Geometry: final body of the model. Coordinates: model frame, mm. A direction names the side the tool comes from. Give positions to 0.01 mm unless a question says otherwise; leave off trailing zeros. Order: outer loops, then holes, each group sorted by start corner. A loop starts at its lowest first (then second) coordinate and runs counter-clockwise, first axis right, second up. Notation, with made-up numbers: (44, 27) - (97, 27) arc R13 ccw to (97, 42) - close; hole circle Ø1 at (3, -10.75). An arc over 180 degrees is marked (long way). Use one line per item in the form item = value.
from build123d import *

# Parameters (mm, degrees)
BOSS_EXTRUDE1_DEPTH = 5.08
SKETCH2_R           = 1.778
CUT_EXTRUDE1_DEPTH  = 55.120480412
SKETCH3_W           = 43.18
SKETCH3_H           = 20.32
CUT_EXTRUDE2_DEPTH  = 55.120480412
SKETCH10_R          = 1.524
CUT_EXTRUDE3_DEPTH  = 55.120480412
SKETCH11_W          = 7.62
SKETCH11_H          = 2.54
CUT_EXTRUDE4_DEPTH  = 55.120480412
CUT_EXTRUDE5_DEPTH  = 55.120480412
SKETCH14_R          = 1.905
CUT_EXTRUDE6_DEPTH  = 55.120480412
CHAMFER1_SIZE       = 16.51
CHAMFER3_SIZE       = 16.51
FILLET1_R           = 12.7
FILLET2_R           = 12.7
SKETCH15_W          = 6.35
SKETCH15_H          = 25.4
CUT_EXTRUDE7_DEPTH  = 55.120480412
SKETCH18_W          = 25.4
SKETCH18_H          = 12.7
BOSS_EXTRUDE3_DEPTH = 5.08
SKETCH19_R          = 0.889
CUT_EXTRUDE9_DEPTH  = 69.814783295
FILLET4_R           = 6.35
SKETCH20_W          = 25.4
SKETCH20_H          = 2.54
CUT_EXTRUDE10_DEPTH = 69.814783351
CHAMFER4_SIZE       = 7.62
CHAMFER4_SIZE2      = 4.399409051
FILLET5_R           = 6.35
FILLET6_R           = 6.35


with BuildPart() as part:
    # Sketch1 → Boss-Extrude1 (new body)
    with BuildSketch(Plane(origin=(0, 0, 0), x_dir=(1, 0, 0), z_dir=(0, 1, 0))):
        Polygon((-38.1, -12.7), (-38.1, 38.1), (38.1, 38.1), (38.1, -12.7), (19.05, -12.7), (19.05, -38.1), (-19.05, -38.1), (-19.05, -12.7), align=None)
    extrude(amount=BOSS_EXTRUDE1_DEPTH)

    # Sketch2 → Cut-Extrude1 (cut, through all)
    with BuildSketch(Plane(origin=(0, 5.08, 0), x_dir=(1, 0, 0), z_dir=(0, 1, 0))):
        with Locations(Location((-22.225, 29.972, 0), (0, 0, 270))):
            Circle(SKETCH2_R)
        with Locations(Location((22.225, 29.972, 0), (0, 0, 90))):
            Circle(SKETCH2_R)
    extrude(amount=-CUT_EXTRUDE1_DEPTH, mode=Mode.SUBTRACT)

    # Sketch3 → Cut-Extrude2 (cut, through all)
    with BuildSketch(Plane(origin=(0, 5.08, 0), x_dir=(1, 0, 0), z_dir=(0, 1, 0))):
        with Locations((0, 9.652)):
            Rectangle(SKETCH3_W, SKETCH3_H)
    extrude(amount=-CUT_EXTRUDE2_DEPTH, mode=Mode.SUBTRACT)

    # Sketch10 → Cut-Extrude3 (cut, through all)
    with BuildSketch(Plane.XZ):
        with Locations(Location((25.4, -14.859, 0), (0, 0, 270))):
            Circle(SKETCH10_R)
        with Locations(Location((25.4, -4.445, 0), (0, 0, 90))):
            Circle(SKETCH10_R)
        with Locations(Location((-25.4, -14.859, 0), (0, 0, 90))):
            Circle(SKETCH10_R)
        with Locations(Location((-25.4, -4.445, 0), (0, 0, 270))):
            Circle(SKETCH10_R)
    extrude(amount=-CUT_EXTRUDE3_DEPTH, mode=Mode.SUBTRACT)

    # Sketch11 → Cut-Extrude4 (cut, through all)
    with BuildSketch(Plane.XZ):
        with Locations((25.4, -9.652)):
            Rectangle(SKETCH11_W, SKETCH11_H)
        with Locations((-25.4, -9.652)):
            Rectangle(SKETCH11_W, SKETCH11_H)
    extrude(amount=-CUT_EXTRUDE4_DEPTH, mode=Mode.SUBTRACT)

    # Sketch12 → Cut-Extrude5 (cut, through all)
    with BuildSketch(Plane.XZ):
        Polygon((22.225, -38.1), (0, -30.48), (-22.225, -38.1), align=None)
    extrude(amount=-CUT_EXTRUDE5_DEPTH, mode=Mode.SUBTRACT)

    # Sketch14 → Cut-Extrude6 (cut, through all)
    with BuildSketch(Plane.XZ):
        with Locations(Location((31.75, 3.048, 0), (0, 0, 270))):
            Circle(SKETCH14_R)
        with Locations(Location((31.75, -22.352, 0), (0, 0, 90))):
            Circle(SKETCH14_R)
        with Locations(Location((-31.75, 3.048, 0), (0, 0, 90))):
            Circle(SKETCH14_R)
        with Locations(Location((-31.75, -22.352, 0), (0, 0, 270))):
            Circle(SKETCH14_R)
    extrude(amount=-CUT_EXTRUDE6_DEPTH, mode=Mode.SUBTRACT)

    # Chamfer1
    # the kernel refuses this chamfer: 16.51 mm, written as the material it takes off along each edge
    with BuildSketch(Plane(origin=(38.1, -42.458486131, -38.1), x_dir=(0.027495876610586233, 0, 0.9996219169112966), z_dir=(0, 1, 0))) as chamfer1_piece_1:
        Polygon((CHAMFER1_SIZE * 0.999621916911, -CHAMFER1_SIZE * 0.0274958766106), (-CHAMFER1_SIZE * 0.0274958766106, -CHAMFER1_SIZE * 0.999621916911), (0, 0), align=None)
    extrude(amount=89.996972263, mode=Mode.SUBTRACT)

    # Chamfer3
    # the kernel refuses this chamfer: 16.51 mm, written as the material it takes off along each edge
    with BuildSketch(Plane(origin=(-38.1, -42.458486131, -38.1), x_dir=(-0.02749587661058624, 0, 0.9996219169112966), z_dir=(0, 1, 0))) as chamfer3_piece_1:
        Polygon((CHAMFER3_SIZE * 0.999621916911, CHAMFER3_SIZE * 0.0274958766106), (-CHAMFER3_SIZE * 0.0274958766106, CHAMFER3_SIZE * 0.999621916911), (0, 0), align=None)
    extrude(amount=89.996972263, mode=Mode.SUBTRACT)

    # Fillet1
    fillet1_edges = [part.edges().sort_by_distance(p)[0] for p in [
        (21.75212766, 2.54, -37.93787234),
        (-21.75212766, 2.54, -37.93787234),
    ]]
    fillet(fillet1_edges, radius=FILLET1_R)

    # Fillet2
    fillet2_edges = [part.edges().sort_by_distance(p)[0] for p in [
        (38.1, 2.54, 12.7),
        (-38.1, 2.54, 12.7),
    ]]
    fillet(fillet2_edges, radius=FILLET2_R)

    # Sketch15 → Cut-Extrude7 (cut, through all)
    with BuildSketch(Plane.XZ):
        with Locations((15.875, 25.4)):
            Rectangle(SKETCH15_W, SKETCH15_H)
        with Locations((-15.875, 25.4)):
            Rectangle(SKETCH15_W, SKETCH15_H)
    extrude(amount=-CUT_EXTRUDE7_DEPTH, mode=Mode.SUBTRACT)

    # Sketch18 → Boss-Extrude3 (add)
    with BuildSketch(Plane(origin=(12.7, 0, 0), x_dir=(0, 0, -1), z_dir=(1, 0, 0))):
        with Locations((-25.4, 6.35)):
            Rectangle(SKETCH18_W, SKETCH18_H)
    extrude(amount=BOSS_EXTRUDE3_DEPTH)

    # Sketch19 → Cut-Extrude9 (cut, through all)
    with BuildSketch(Plane(origin=(17.78, 0, 0), x_dir=(0, 0, -1), z_dir=(1, 0, 0))):
        with Locations((-16.51, 6.35)):
            Circle(SKETCH19_R)
        with Locations((-21.59, 6.35)):
            Circle(SKETCH19_R)
    extrude(amount=-CUT_EXTRUDE9_DEPTH, mode=Mode.SUBTRACT)

    # Fillet4
    # the kernel refuses this fillet: 6.35 mm, written as the material it adds along each edge
    with BuildSketch(Plane(origin=(12.7, 5.08, 12.7), x_dir=(-1, 0, 0), z_dir=(0, 0, 1))) as fillet4_piece_1_section:
        with BuildLine():
            CenterArc((FILLET4_R, -FILLET4_R), FILLET4_R, 90, 90)
            Line((0, -FILLET4_R), (0, 0))
            Line((0, 0), (FILLET4_R, 0))
        make_face()
    fillet4_piece_1 = extrude(amount=25.4, mode=Mode.PRIVATE)
    fillet4_piece_1 = fillet4_piece_1 - Plane(origin=(11.255700074, 6.35, 16.51), x_dir=(0, 0, -1), z_dir=(1, 0, 0)) * Cylinder(0.889, 77, mode=Mode.PRIVATE)
    fillet4_piece_1 = fillet4_piece_1 - Plane(origin=(11.255700074, 6.35, 21.59), x_dir=(0, 0, -1), z_dir=(1, 0, 0)) * Cylinder(0.889, 77, mode=Mode.PRIVATE)
    add(fillet4_piece_1)

    # Sketch20 → Cut-Extrude10 (cut, through all)
    with BuildSketch(Plane(origin=(17.78, 0, 0), x_dir=(0, 0, -1), z_dir=(1, 0, 0))):
        with Locations((-25.4, 11.43)):
            Rectangle(SKETCH20_W, SKETCH20_H)
    extrude(amount=-CUT_EXTRUDE10_DEPTH, mode=Mode.SUBTRACT)

    # Chamfer4
    chamfer4_edges = [part.edges().sort_by_distance(p)[0] for p in [
        (15.175851973, 10.16, 38.1),
    ]]
    chamfer4_side = [part.faces().sort_by_distance(p)[0] for p in [
        (15.175851973, 10.16, 25.4),
    ]]
    chamfer(chamfer4_edges, length=CHAMFER4_SIZE, length2=CHAMFER4_SIZE2, reference=chamfer4_side[0])

    # Fillet5
    fillet5_edges = [part.edges().sort_by_distance(p)[0] for p in [
        (15.175851973, 10.16, 30.48),
    ]]
    fillet(fillet5_edges, radius=FILLET5_R)

    # Fillet6
    # the kernel refuses this fillet: 6.35 mm, written as the material it takes off along each edge
    with BuildSketch(Plane(origin=(33.334259867, 10.16, 12.7), x_dir=(0, 0, 1), z_dir=(-1, 0, 0))) as fillet6_piece_1:
        with BuildLine():
            CenterArc((6.221703947, -6.35), FILLET6_R, 90, 78.463040967)
            Line((0, -5.08), (-0.124434079, -5.0546))
            ThreePointArc((-0.124434079, -5.0546), (-0.127, -2.54), (-0.127, 0))
            Line((-0.127, 0), (0, 0.127))
            Line((0, 0.127), (6.221703947, 0.127))
            Line((6.221703947, 0.127), (6.221703947, 0))
        make_face()
    extrude(amount=36.316815787, mode=Mode.SUBTRACT)


solid = part.part
(1) Reachability of faces 1 (the face through (7.23, 2.5, -32.96)), 2 (the face through (2, 3, 38.1)), 3 (the face through (-19, 3, 12.7)), 4 (the face through (25, 3, -10.922)) from +Z, -Z, +X, -X, +Y, -Y: full face, straight path, thin tool, end or side. Return the list, or none.
Computed values:
face_1 = -Z, +Y, -Y
face_2 = +Z, +X, -X, +Y, -Y
face_3 = +Z, -X, +Y, -Y
face_4 = +Y, -Y
(2) Cut plane A-A on x = -6. Output: boundary loops of the cut face in (y, z), plus the area to 3 significant figures.
Computed values:
outline = (0, -32.54) - (5.08, -32.54) - (5.08, -19.81) - (0, -19.81) - close; (0, 0.51) - (5.08, 0.51) - (5.08, 38.1) - (0, 38.1) - close
area = 256 mm²
(3) Cut plane D-D on y = 2.5. Give the number of separate pieces and of enclosed holes in the cut face, plus the area to 3 significant figures.
Computed values:
separate_pieces = 1
enclosed_holes = 11
area = 3,100 mm²
(4) Cut plane C-C on x = -31.75. Output: boundary loops of the cut face in (y, z).
Computed values:
outline = (0, -27.94) - (5.08, -27.94) - (5.08, -24.26) - (0, -24.26) - close; (0, -20.45) - (5.08, -20.45) - (5.08, 1.14) - (0, 1.14) - close; (0, 4.95) - (5.08, 4.95) - (5.08, 11) - (0, 11) - close
(5) Pull-direction query (Z, two-part tool) for faces 5 (the face through (14.51, 7.51, 35.07)), 6 (the face through (25, 3, -8.382)), 7 (the face through (1, 5.08, 9)); classes: released by +Z, released by -Z, zero draft, split by the parting line, or undercut.
Computed values:
face_5 = released by +Z
face_6 = undercut
face_7 = zero draft
(6) Contact query for flat-ended pins moving along their axis: pin 1 Ø4.5 at (x, z) = (31.75, -22.352) entering from +Y; pin 2 Ø2.5 at (x, y) = (4.5, 3) entering from -Z; pin 3 Ø6 at (x, y) = (0.5, 2.5) entering from -Z; pin 4 Ø2 at (y, z) = (4, 0.5) entering from -X. Output: stop coordinate, or through.
Computed values:
pin_1 = 5.08
pin_2 = -32.45
pin_3 = -31.68
pin_4 = -38.1
(7) Cut plane B-B on z = 23.5. Output: boundary loops of the cut face in (x, y), plus the area to 3 significant figures.
Computed values:
outline = (-12.7, 0) - (17.78, 0) - (17.78, 10.16) - (12.57, 10.16) arc R6.35 cw to (6.35, 5.08) - (-12.7, 5.08) - close
area = 189 mm²
(8) Ray query, line 1 along Z through (x, y) = (-22.5, 1.5); line 2 along Z through (x, y) = (-30.5, 5); line 3 along Y through (x, z) = (10.5, 21.59). Return the intervals inside material, ascending.
Computed values:
line_1 = -35.37 to -31.73, -28.22 to -10.92, -8.38 to 12.7
line_2 = -29.19 to -23.79, -20.91 to 1.61, 4.49 to 11.63
line_3 = 0 to 5.46
